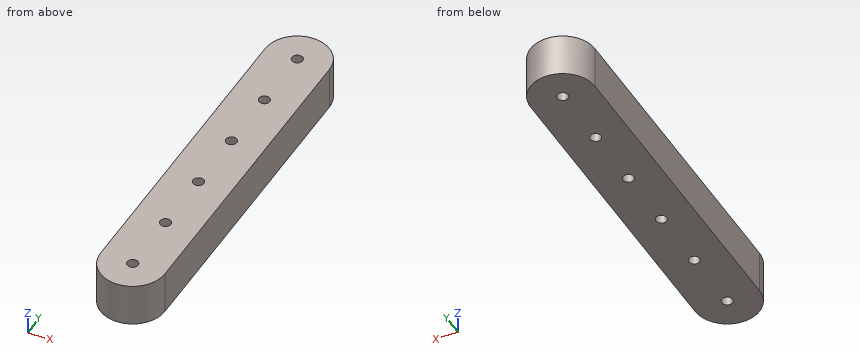
Autodesk Inventor part; units mm, degrees
ref_plane "YZ Plane" through (0, 0, 0) normal (1, 0, 0) x (0, 1, 0)
ref_plane "XZ Plane" through (0, 0, 0) normal (0, 1, 0) x (-1, 0, 0)
ref_plane "XY Plane" through (0, 0, 0) normal (0, 0, 1) x (1, 0, 0)
sketch "Sketch1" plane through (0, 0, 0) normal (0, 0, 1) x (1, 0, 0)
  line L0 (0, -63.5) -> (0, 63.5) construction
  line L1 (12.7, -63.5) -> (12.7, 63.5)
  line L2 (-12.7, 63.5) -> (-12.7, -63.5)
  arc A0 (-12.7, -63.5) -> (12.7, -63.5) centre (0, -63.5) ccw
  arc A1 (12.7, 63.5) -> (-12.7, 63.5) centre (0, 63.5) ccw
  point P0 (0, 0)
  point P1 (0, 38.1)
  point P2 (0, 12.7)
  point P3 (0, -12.7)
  point P4 (0, -38.1)
  dimension "d0" = 63.5
  dimension "d1" = 25.4
  dimension "d2" = 25.4
  dimension "d3" = 25.4
  dimension "d4" = 25.4
  dimension "d5" = 25.4
extrude "Extrusion1" add sketch "Sketch1" along normal blind 17.145
hole "Hole1" at (0, 38.1, 0) at (0, 12.7, 0) at (0, -12.7, 0) at (0, -38.1, 0) at (0, -63.5, 0) at (0, 63.5, 0) direction (0, 0, 1) diameter 4.318 end through all
properties part number "Motor Bracket Seperator" material "PET Plastic"
For this review, take the finished solid that the model builds, in its own axes (mm). Give positions to 0.01 mm unless a question says otherwise; leave off trailing zeros. Loops run counter-clockwise (first coordinate to the right, second up) from the corner with the lowest first, then second, coordinate; pieces in that order, holes last. Notation, with made-up numbers: M 15.25,16 L 25.25,16 A13 cw 25.25,20 Z; hole C 43,9.25 d4. An arc over 180 degrees is marked long. Put each result on its own line as item: value. Start each with the question number.
(1) Wall thickness on L1, parallel to X at y = 12.7, z = 13.5; L2, parallel to X at y = -38.5, z = 5.75; L3, parallel to Y at x = -7.75, z = 3.25: over which ranges is each line inside the solid? List them lowest first.
(2) For pin 1 (4 mm diameter, centred on x = 0, y = 12.7, fed in from +Z); pin 2 (3 mm diameter, centred on x = 7.5, z = 3.5, fed in from -Y); pin 3 (1 mm diameter, centred on x = -5, z = 4.5, fed in from +Y); pin 4 (2 mm diameter, centred on x = -7.5, z = 3.5, fed in from -Y), all flat-tipped, find the tip position at first contact; note any pin that passes through.
(3) Add section D-D, the plane y = 38.5. Write out the cut boundary in (x, z) (3 decimals), then the cut area to 3 significant figures.
(4) Add section B-B, the plane y = 12.7. Write out the cut boundary in (x, z) (3 decimals).
(5) Add section A-A, the plane x = 0. Write out the cut boundary in (y, z) (3 decimals).
(6) Add section C-C, the plane z = 10.5. Write out the cut boundary in (x, y).
Result:
1. L1: x = -12.7 to -2.16, 2.16 to 12.7
1. L2: x = -12.7 to -2.12, 2.12 to 12.7
1. L3: y = -73.56 to 73.56
2. pin 1: passes through
2. pin 2: stops at y = -74.69
2. pin 3: stops at y = 75.38
2. pin 4: stops at y = -74.41
3. outline: M -12.7,0 L -2.122,0 L -2.122,17.145 L -12.7,17.145 Z; M 2.122,0 L 12.7,0 L 12.7,17.145 L 2.122,17.145 Z
3. area: 363 mm^2
4. outline: M -12.7,0 L -2.159,0 L -2.159,17.145 L -12.7,17.145 Z; M 2.159,0 L 12.7,0 L 12.7,17.145 L 2.159,17.145 Z
5. outline: M -76.2,0 L -65.659,0 L -65.659,17.145 L -76.2,17.145 Z; M -61.341,0 L -40.259,0 L -40.259,17.145 L -61.341,17.145 Z; M -35.941,0 L -14.859,0 L -14.859,17.145 L -35.941,17.145 Z; M -10.541,0 L 10.541,0 L 10.541,17.145 L -10.541,17.145 Z; M 14.859,0 L 35.941,0 L 35.941,17.145 L 14.859,17.145 Z; M 40.259,0 L 61.341,0 L 61.341,17.145 L 40.259,17.145 Z; M 65.659,0 L 76.2,0 L 76.2,17.145 L 65.659,17.145 Z
6. outline: M -12.7,-63.5 A12.7 ccw 12.7,-63.5 L 12.7,63.5 A12.7 ccw -12.7,63.5 Z; hole C 0,-63.5 d4.32; hole C 0,-38.1 d4.32; hole C 0,-12.7 d4.32; hole C 0,12.7 d4.32; hole C 0,38.1 d4.32; hole C 0,63.5 d4.32
